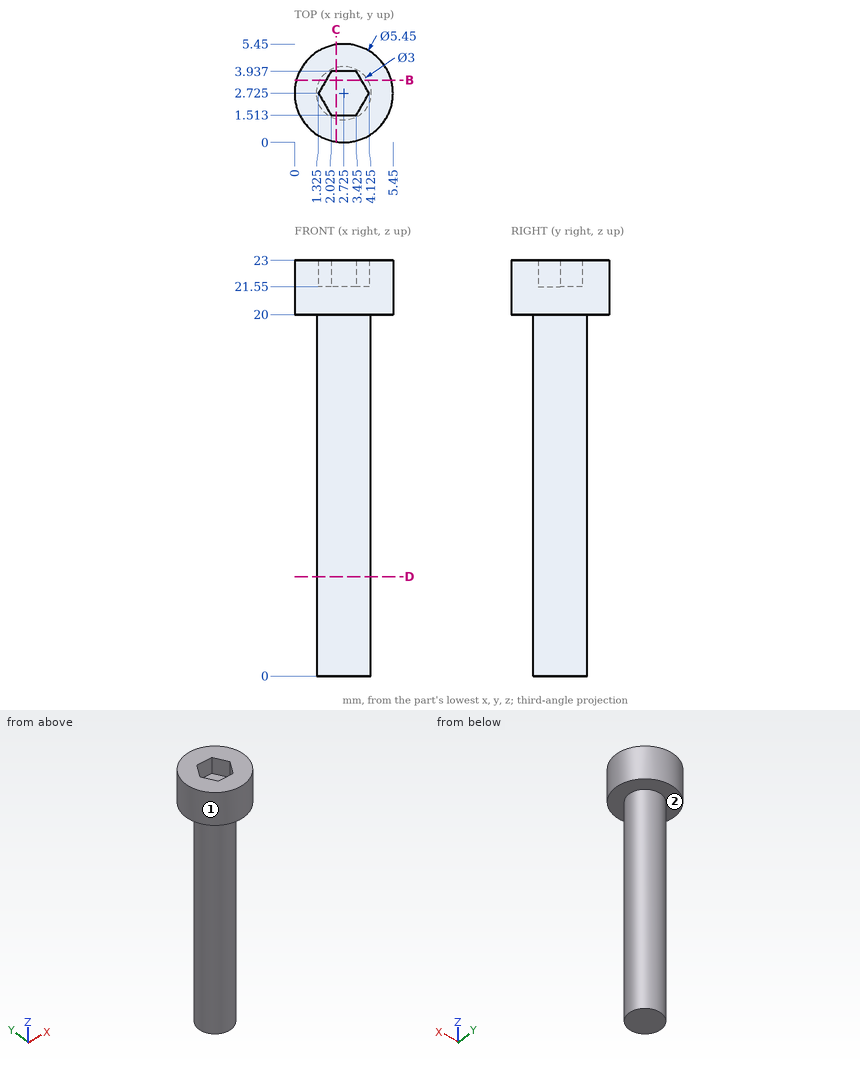
Answer from the drawing. Dimensions are ordinates in mm from the lowest x, y and z of the part. A direction names the side the tool comes from. Round coordinates to 2 decimals unless told otherwise and drop trailing zeros. Order: outer loops, then holes, each group sorted by start corner. A loop starts at its lowest first (then second) coordinate and runs counter-clockwise, first axis right, second up.
1) The part is cut by section D-D on z = 5.5. Write down the section's boundary in (x, y) (1 decimal).
2) Flat-ended cylindrical pins translate along their axes: pin 1 (3 mm diameter, centred on y = 1, z = 10, fed in from -X); pin 2 (1 mm diameter, centred on y = 1, z = 8, fed in from +X); pin 3 (3 mm diameter, centred on x = 1.5, z = 12.5, fed in from +Y) (3 decimals). Find the tip coordinate at first contact, or state that the pin passes through.
3) Straight lines are drawn through the part: L1, parallel to Z at x = 4, y = 0.9; L2, parallel to Y at x = 2.8, z = 12; L3, parallel to Y at x = 3.6, z = 7.25 (1 decimal). For each, find the intervals that lie inside material, in ascending order.
4) For the marked faces 1 and 2, determine the directions among +Z, -Z, +X, -X, +Y, -Y from which every point of the face is accessible in a straight line to the end or side of a thin tool.
5) The part is cut by section C-C on x = 2.3. Write down the section's boundary in (y, z).
6) The part is cut by section B-B on y = 3.45. Write down the section's boundary in (x, z).
Resolved:
1. outline: circle Ø3 at (2.7, 2.7)
2. pin 1: stops at x = 1.24
2. pin 2: stops at x = 3.59
2. pin 3: stops at y = 4.225
3. L1: z = 20 to 23
3. L2: y = 1.23 to 4.22
3. L3: y = 1.5 to 3.9
4. face 1: +Z, -Z
4. face 2: -Z
5. outline: (0.03, 20) - (1.29, 20) - (1.29, 0) - (4.16, 0) - (4.16, 20) - (5.42, 20) - (5.42, 23) - (3.94, 23) - (3.94, 21.55) - (1.51, 21.55) - (1.51, 23) - (0.03, 23) - close
6. outline: (0.1, 20) - (1.41, 20) - (1.41, 0) - (4.04, 0) - (4.04, 20) - (5.35, 20) - (5.35, 23) - (3.71, 23) - (3.71, 21.55) - (1.74, 21.55) - (1.74, 23) - (0.1, 23) - close
